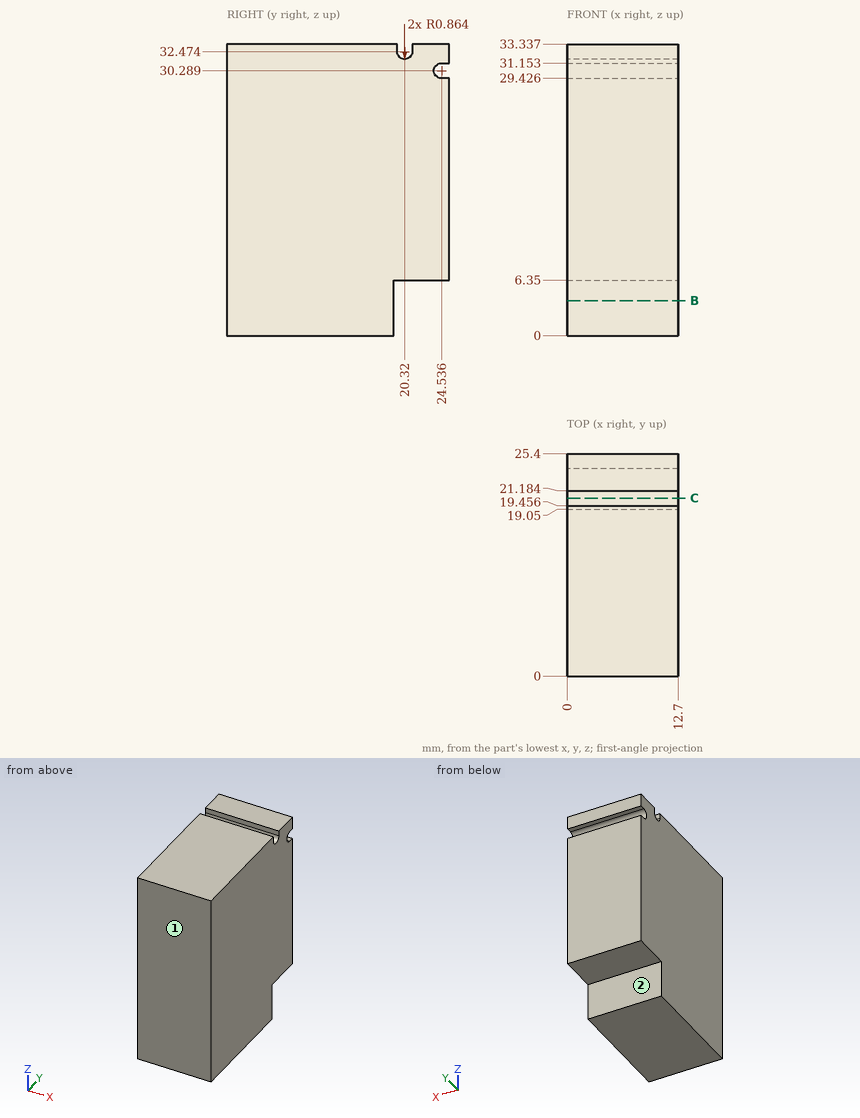
Source: three-view drawing plus pictorial views. Frame: mm from the lowest corner of the part. A direction names the side the tool comes from. Coordinates: 2 decimals unless noted, no trailing zeros. Loops run counter-clockwise (first coordinate to the right, second up) from the corner with the lowest first, then second, coordinate; pieces in that order, holes last. Notation, with made-up numbers: (86, 56) -> (107, 56) arc R16 cw to (107, 83) -> close; hole circle Ø2 at (47, 69.25). An arc over 180 degrees is marked (long way). Write each question's results on one line, items separated by ' | '. Start each with the question number.
Q1. Reachability of the marked faces 1 and 2 from +Z, -Z, +X, -X, +Y, -Y: full face, straight path, thin tool, end or side. Return the list, or none.
Q2. Section B-B, the plane z = 4. Return the cut outline in (x, y), plus the area to 3 significant figures.
Q3. Pin query (flat end, axial travel): pin 1 (0.7 mm diameter, centred on x = 5.5, y = 25, fed in from -Z); pin 2 (1.9 mm diameter, centred on x = 6, z = 3.5, fed in from +Y). Return the tip coordinate at first contact, or that it passes through.
Q4. Ray query, line 1 (Z direction, x = 5.75, y = 24.5); line 2 (Z direction, x = 9.25, y = 23); line 3 (Y direction, x = 4.75, z = 5). Return the intervals inside material, ascending. Write a range as from..to.
Q5. Section C-C, the plane y = 20.32. Return the cut outline in (x, z), plus the area to 3 significant figures.
Found:
1) face 1: +Z, -Z, +X, -X, -Y | face 2: -Z, +X, -X, +Y
2) outline: (0, 0) -> (12.7, 0) -> (12.7, 19.05) -> (0, 19.05) -> close | area: 242 mm2
3) pin 1: z = 6.35 | pin 2: y = 19.05
4) line 1: 6.35..29.43, 31.15..33.34 | line 2: 6.35..33.34 | line 3: 0..19.05
5) outline: (0, 6.35) -> (12.7, 6.35) -> (12.7, 31.61) -> (0, 31.61) -> close | area: 321 mm2
